from build123d import *

# Parameters (mm, degrees)
SKETCH1_W     = 2.5
SKETCH1_H     = 4
CHAMFER1_SIZE = 0.1


with BuildPart() as part:
    # Sketch1 → Revolve1 (revolve)
    with BuildSketch(Plane(origin=(0, 0, 0), x_dir=(0, 0, -1), z_dir=(1, 0, 0))):
        with Locations((6.25, 0)):
            Rectangle(SKETCH1_W, SKETCH1_H)
    revolve(axis=Axis((0, 2, 0), (0, -1, 0)))

    # Sketch3 → Cut-Revolve2 (revolve, cut)
    with BuildSketch(Plane(origin=(0, 0, 0), x_dir=(0, 0, -1), z_dir=(1, 0, 0))):
        Polygon((6.55, 1.8), (6.75, 1.6), (6.75, 2), (5.75, 2), (5.75, 1.6), (5.95, 1.8), align=None)
    cut_revolve2 = revolve(axis=Axis((0, 2, 0), (0, -1, 0)), mode=Mode.SUBTRACT)

    # Mirror1: Cut-Revolve2 across plane
    add(cut_revolve2.mirror(Plane.ZX), mode=Mode.SUBTRACT)

    # Chamfer1
    chamfer1_edges = [part.edges().sort_by_distance(p)[0] for p in [
        (0, 2, 6.75),
        (0, 2, 5.75),
        (0, -2, 6.75),
        (0, -2, 5.75),
        (0, 2, 7.5),
        (0, -2, 7.5),
        (0, -2, 5),
        (0, 2, 5),
    ]]
    chamfer(chamfer1_edges, length=CHAMFER1_SIZE)


solid = part.part
Can you work these out from the model? Positions are in its coordinate system, mm. A direction names the side the tool comes from. Coordinates: 2 decimals unless noted, no trailing zeros. Loops run counter-clockwise (first coordinate to the right, second up) from the corner with the lowest first, then second, coordinate; pieces in that order, holes last. Notation, with made-up numbers: (-10.75, 0) - (37.25, 0) arc R14 cw to (37.25, 20) - close; hole circle Ø10 at (28.5, 14). An arc over 180 degrees is marked (long way). Put each result on its own line as item: value. Start each with the question number.
Item 1: Which directions (+Z, -Z, +X, -X, +Y, -Y) give clear straight access to the entire face, cutting with the end or side of a thin tool? Please do faces 4 (the face through (-6, 1.8, 2)), 5 (the face through (-6, -1.8, 2)).
Item 2: For pin 1 (2 mm diameter, centred on x = 2.5, y = 1, fed in from +Z); pin 2 (1.5 mm diameter, centred on x = -5, y = 1.5, fed in from +Z); pin 3 (1.5 mm diameter, centred on x = 5, y = 0.5, fed in from -Z), each with a flat end and sliding along its axis, tell me the tip position at first contact or that it passes through.
Item 3: If I drill on line 1 along X through (y, z) = (1.85, -3.5); line 2 along X through (y, z) = (0.7, 0); line 3 along X through (y, z) = (0.6, -5.5), over which ranges is the centre line in solid material (lowest first)?
Item 4: Suppose I cut it at A-A (y = 0.55). Please give me the cut outline in (x, z), and give its area (3 significant figures).
Item 5: If we mould it in two halves opening along X, with no side actions, what happens to faces 1 (the face through (-5, -2, 5)), 2 (the face through (0.33, 0.027, 7.493)), 3 (the face through (-4.88, 0.03, 1.08))? For each: +X half, -X half, draft (parallel to the pull), parting line (faces both ways), or undercut.
Here are the results:
1. face 4: +Y
1. face 5: -Y
2. pin 1: z = 7.35
2. pin 2: z = 6.18
2. pin 3: z = -6.18
3. line 1: -6.63 to -5.77, -4.56 to -3.57, 3.57 to 4.56, 5.77 to 6.63
3. line 2: -7.5 to -5, 5 to 7.5
3. line 3: -5.1 to 5.1
4. outline: circle Ø15 at (0, 0); hole circle Ø10 at (0, 0)
4. area: 98.2 mm²
5. face 1: draft
5. face 2: parting line
5. face 3: undercut
